CAD build for the part. Positions are in the model's coordinates, mm. Face numbers are marked on the shaded views. Give positions to 0.01 mm unless a question says otherwise; leave off trailing zeros. Loops run counter-clockwise (first coordinate to the right, second up) from the corner with the lowest first, then second, coordinate; pieces in that order, holes last. Notation, with made-up numbers: M -4,0 L 30,0 A17 cw 30,23 Z; hole C 15.5,87 d8. An arc over 180 degrees is marked long. Answer as CSV lines item,"result".
from build123d import *

# Parameters (mm, degrees)
SKETCH_1_W          = 20
SKETCH_1_H          = 10
SKETCH_1_W_2        = 17
SKETCH_1_H_2        = 7
EXTRUDE_1_DEPTH     = 150
SKETCH_2_R          = 2.15
SKETCH_2_R_2        = 2.5
CUT_EXTRUDE_1_DEPTH = 151.665191733
SKETCH_3_R          = 2.15
CUT_EXTRUDE_2_DEPTH = 152.410039297


with BuildPart() as part:
    # ｽｹｯﾁ1 → 押し出し-薄板1 (new body)
    with BuildSketch(Plane.XY):
        Rectangle(SKETCH_1_W, SKETCH_1_H)
        Rectangle(SKETCH_1_W_2, SKETCH_1_H_2, mode=Mode.SUBTRACT)
    extrude(amount=EXTRUDE_1_DEPTH)

    # ｽｹｯﾁ2 → ｶｯﾄ - 押し出し1 (cut, through all)
    with BuildSketch(Plane(origin=(0, 5, 0), x_dir=(1, 0, 0), z_dir=(0, 1, 0))):
        with Locations(Location((5, -142, 0), (0, 0, 270))):
            Circle(SKETCH_2_R)
        with Locations(Location((-5, -142, 0), (0, 0, 270))):
            Circle(SKETCH_2_R)
        with Locations(Location((5, -8, 0), (0, 0, 270))):
            Circle(SKETCH_2_R)
        with Locations(Location((-5, -8, 0), (0, 0, 270))):
            Circle(SKETCH_2_R)
        with Locations(Location((0, -35, 0), (0, 0, 270))):
            Circle(SKETCH_2_R_2)
        with Locations(Location((0, -115, 0), (0, 0, 270))):
            Circle(SKETCH_2_R_2)
    extrude(amount=-CUT_EXTRUDE_1_DEPTH, mode=Mode.SUBTRACT)

    # ｽｹｯﾁ3 → ｶｯﾄ - 押し出し2 (cut, through all)
    with BuildSketch(Plane(origin=(10, 0, 0), x_dir=(0, 0, -1), z_dir=(1, 0, 0))):
        with Locations((-60, 0)):
            Circle(SKETCH_3_R)
        with Locations(Location((-90, 0, 0), (0, 0, 90))):
            Circle(SKETCH_3_R)
    extrude(amount=-CUT_EXTRUDE_2_DEPTH, mode=Mode.SUBTRACT)


solid = part.part
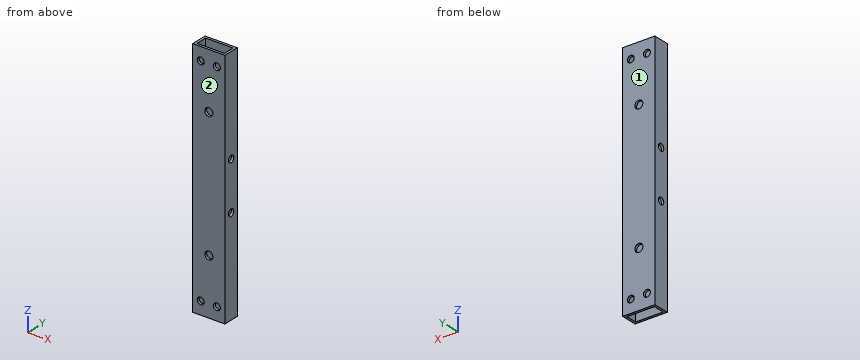
1) Band-saw the part on A-A on x = 0. Give the cut face in (y, z), and give its area (3 significant figures).
Answer below:
outline,"M -5,0 L -3.5,0 L -3.5,32.5 L -5,32.5 Z; M -5,37.5 L -3.5,37.5 L -3.5,112.5 L -5,112.5 Z; M -5,117.5 L -3.5,117.5 L -3.5,150 L -5,150 Z; M 3.5,0 L 5,0 L 5,32.5 L 3.5,32.5 Z; M 3.5,37.5 L 5,37.5 L 5,112.5 L 3.5,112.5 Z; M 3.5,117.5 L 5,117.5 L 5,150 L 3.5,150 Z"
area,"420 mm^2"
2) Mould opens along Y. For the marked faces 1 and 2 say: +Y half, -Y half, draft (parallel to the pull), parting line (faces both ways), or undercut.
Answer below:
face 1,"+Y half"
face 2,"-Y half"
3) Band-saw the part on C-C on y = 0. Give the cut face in (x, z), and give its area (3 significant figures).
Answer below:
outline,"M -10,0 L -8.5,0 L -8.5,57.85 L -10,57.85 Z; M -10,62.15 L -8.5,62.15 L -8.5,87.85 L -10,87.85 Z; M -10,92.15 L -8.5,92.15 L -8.5,150 L -10,150 Z; M 8.5,0 L 10,0 L 10,57.85 L 8.5,57.85 Z; M 8.5,62.15 L 10,62.15 L 10,87.85 L 8.5,87.85 Z; M 8.5,92.15 L 10,92.15 L 10,150 L 8.5,150 Z"
area,"424 mm^2"
4) Flat gauge pin, fed straight in: pin 1 (2.5 mm diameter, centred on y = 0, z = 90, fed in from -X). Where does the tip first touch, or does it go through?
Answer below:
pin 1,"passes through"
5) Band-saw the part on D-D on z = 60. Give the cut face in (x, y).
Answer below:
outline,"M -10,-5 L 10,-5 L 10,-2.15 L 8.5,-2.15 L 8.5,-3.5 L -8.5,-3.5 L -8.5,-2.15 L -10,-2.15 Z; M -10,2.15 L -8.5,2.15 L -8.5,3.5 L 8.5,3.5 L 8.5,2.15 L 10,2.15 L 10,5 L -10,5 Z"
6) Band-saw the part on B-B on z = 8. Give the cut face in (x, y).
Answer below:
outline,"M -10,-5 L -7.15,-5 L -7.15,-3.5 L -8.5,-3.5 L -8.5,3.5 L -7.15,3.5 L -7.15,5 L -10,5 Z; M -2.85,-5 L 2.85,-5 L 2.85,-3.5 L -2.85,-3.5 Z; M -2.85,3.5 L 2.85,3.5 L 2.85,5 L -2.85,5 Z; M 7.15,-5 L 10,-5 L 10,5 L 7.15,5 L 7.15,3.5 L 8.5,3.5 L 8.5,-3.5 L 7.15,-3.5 Z"
7) Drill centre lines: line 1 (X direction, y = 4.6, z = 142); line 2 (X direction, y = -4.25, z = 115); line 3 (X direction, y = -1.25, z = 27). Where is each one in solid material? Low to high. Write a range as from..to.
Answer below:
line 1,"x = -10..-7.15, -2.85..2.85, 7.15..10"
line 2,"x = -10..-2.5, 2.5..10"
line 3,"x = -10..-8.5, 8.5..10"
